```python
from build123d import *

# Parameters (mm, degrees)
SKETCH1_R           = 66.675
BOSS_EXTRUDE1_DEPTH = 127.0635
DOME1_FACE_RADIUS   = 66.675
DOME1_HEIGHT        = 66.675
SKETCH5_R           = 20.255
BOSS_EXTRUDE2_DEPTH = 16.51
CHAMFER1_SIZE       = 2.54
FILLET1_R           = 6.35


with BuildPart() as part:
    # Sketch1 → Boss-Extrude1 (new body, symmetric)
    with BuildSketch(Plane(origin=(0, 0, 0), x_dir=(1, 0, 0), z_dir=(0, 1, 0))):
        Circle(SKETCH1_R)
    extrude(amount=BOSS_EXTRUDE1_DEPTH, both=True)

    # Dome1: a dome of height H over a round flat face of radius A is a cap of a sphere of radius (A * A + H * H) / (2 * H)
    dome1_r = (DOME1_FACE_RADIUS * DOME1_FACE_RADIUS + DOME1_HEIGHT * DOME1_HEIGHT) / (2 * DOME1_HEIGHT)
    dome1_base = Plane((0, 127.0635, 0), z_dir=(0, 1, 0))
    with Locations(dome1_base.offset(DOME1_HEIGHT - dome1_r)):
        dome1_ball = Sphere(dome1_r, mode=Mode.PRIVATE)
    add(split(dome1_ball, bisect_by=dome1_base, keep=Keep.TOP, mode=Mode.PRIVATE))

    # Sketch5 → Boss-Extrude2 (add, symmetric)
    with BuildSketch(Plane(origin=(0, 193.7385, 0), x_dir=(1, 0, 0), z_dir=(0, 1, 0))):
        Circle(SKETCH5_R)
    extrude(amount=BOSS_EXTRUDE2_DEPTH, both=True)

    # Chamfer1
    chamfer1_edges = [part.edges().sort_by_distance(p)[0] for p in [
        (-66.675, -127.0635, 0),
    ]]
    chamfer(chamfer1_edges, length=CHAMFER1_SIZE)

    # Fillet1
    fillet1_edges = [part.edges().sort_by_distance(p)[0] for p in [
        (-14.322447853, 190.587437221, -14.322447853),
    ]]
    fillet(fillet1_edges, radius=FILLET1_R)


solid = part.part
```
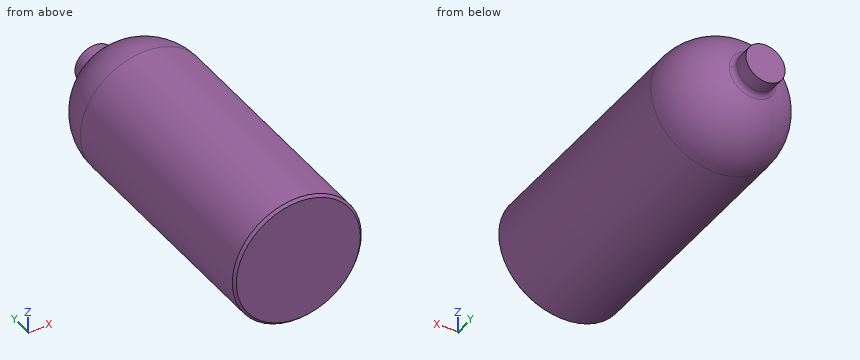
The model under review builds one solid part; all positions refer to its coordinate system, in mm. Coordinates: 2 decimals unless noted, no trailing zeros. Write each loop counter-clockwise with the first axis right and the second up, starting at its lowest first coordinate (ties: lowest second). Pieces come first, ordered by that corner, then holes. Notation, with made-up numbers: (-1, 29) - (57, 29) arc R9 ccw to (57, 39) - close; hole circle Ø4 at (-18.5, -19). An arc over 180 degrees is marked (long way). Write item = value, one per line.
(1) For line 1 (Z direction, x = 3, y = -98.5); line 2 (Y direction, x = -14.5, z = -59); line 3 (Y direction, x = -21.5, z = 15.5), list the stretches that pass through material, from the lowest coordinate up. Write a range as [from, to].
Result sheet:
line_1 = [-66.61, 66.61]
line_2 = [-127.06, 154.53]
line_3 = [-127.06, 188.24]
(2) For P1, Ø1, axis at x = 29.5, z = 38, coming from the +Y side (3 decimals); P2, Ø12, axis at y = 129, z = -1.5, coming from the +X side (3 decimals); P3, Ø6, axis at x = 22.5, y = 17, coming from the -Z side; P4, Ø12, axis at y = 75.5, z = -2, coming from the -X side (3 decimals), all flat-tipped, find the tip position at first contact; note any pin that passes through.
Result sheet:
P1 = 173.745
P2 = 66.675
P3 = -63.76
P4 = -66.675
(3) Consider section A-A, the plane y = 90.5. Give the boundary of the cut face in (x, z) (3 decimals), then the cut area to 3 significant figures.
Result sheet:
outline = circle Ø133.35 at (0, 0)
area = 14,000 mm^2
